from build123d import *

# Parameters (mm, degrees)
BOSS_EXTRUDE1_DEPTH = 4.95
CUT_EXTRUDE1_DEPTH  = 3.45
CUT_EXTRUDE2_REACH  = 63.277
SKETCH3_R           = 0.975
CUT_EXTRUDE3_REACH  = 63.319
SKETCH4_R           = 1.125


with BuildPart() as part:
    # Sketch1 → Boss-Extrude1 (new body)
    with BuildSketch(Plane(origin=(69.394235316, 0, 69.394235316), x_dir=(0.7071067811865475, 0, -0.7071067811865477), z_dir=(0.7071067811865477, 0, 0.7071067811865475))):
        with BuildLine():
            Line((23.501825189, 8.05), (23.501825189, 14.369504832))
            ThreePointArc((23.501825189, 14.369504832), (21.501825189, 17.5), (23.501825189, 20.630495168))
            Line((23.501825189, 20.630495168), (23.501825189, 26.95))
            ThreePointArc((23.501825189, 26.95), (24.380504846, 29.071320344), (26.501825189, 29.95))
            Line((26.501825189, 29.95), (33.522833629, 29.95))
            ThreePointArc((33.522833629, 29.95), (35.951825189, 30.95), (38.38081675, 29.95))
            Line((38.38081675, 29.95), (45.401825189, 29.95))
            ThreePointArc((45.401825189, 29.95), (47.523145533, 29.071320344), (48.401825189, 26.95))
            Line((48.401825189, 26.95), (48.401825189, 20.630495168))
            ThreePointArc((48.401825189, 20.630495168), (50.401825189, 17.5), (48.401825189, 14.369504832))
            Line((48.401825189, 14.369504832), (48.401825189, 8.05))
            ThreePointArc((48.401825189, 8.05), (47.523145533, 5.928679656), (45.401825189, 5.05))
            Line((45.401825189, 5.05), (38.38081675, 5.05))
            ThreePointArc((38.38081675, 5.05), (35.951825189, 4.05), (33.522833629, 5.05))
            Line((33.522833629, 5.05), (26.501825189, 5.05))
            ThreePointArc((26.501825189, 5.05), (24.380504846, 5.928679656), (23.501825189, 8.05))
        make_face()
    extrude(amount=BOSS_EXTRUDE1_DEPTH)

    # Sketch2 → Cut-Extrude1 (cut)
    with BuildSketch(Plane(origin=(72.894413883, 0, 72.894413883), x_dir=(0.7071067811865476, 0, -0.7071067811865476), z_dir=(0.7071067811865476, 0, 0.7071067811865476))):
        with BuildLine():
            Line((38.360144105, 27.95), (46.401825189, 27.95))
            Line((46.401825189, 27.95), (46.401825189, 19.908318916))
            ThreePointArc((46.401825189, 19.908318916), (43.501825189, 17.5), (46.401825189, 15.091681084))
            Line((46.401825189, 15.091681084), (46.401825189, 7.05))
            Line((46.401825189, 7.05), (38.360144105, 7.05))
            ThreePointArc((38.360144105, 7.05), (35.951825189, 5.05), (33.543506273, 7.05))
            Line((33.543506273, 7.05), (25.501825189, 7.05))
            Line((25.501825189, 7.05), (25.501825189, 15.091681084))
            ThreePointArc((25.501825189, 15.091681084), (28.401825189, 17.5), (25.501825189, 19.908318916))
            Line((25.501825189, 19.908318916), (25.501825189, 27.95))
            Line((25.501825189, 27.95), (33.543506273, 27.95))
            ThreePointArc((33.543506273, 27.95), (35.951825189, 29.95), (38.360144105, 27.95))
        make_face()
    extrude(amount=-CUT_EXTRUDE1_DEPTH, mode=Mode.SUBTRACT)

    # Sketch3 → Cut-Extrude2 (cut, up to next)
    with BuildSketch(Plane(origin=(70.454895488, 0, 70.454895488), x_dir=(0.7071067811865475, 0, -0.7071067811865477), z_dir=(0.7071067811865477, 0, 0.7071067811865475)), mode=Mode.PRIVATE) as cut_extrude2_sk1:
        with Locations((35.951825189, 27.5)):
            Circle(SKETCH3_R)
    cut_extrude2_tool1 = extrude(cut_extrude2_sk1.sketch, amount=-CUT_EXTRUDE2_REACH, mode=Mode.PRIVATE) & part.part
    # Sketch3 → Cut-Extrude2 (cut, up to next)
    with BuildSketch(Plane(origin=(70.454895488, 0, 70.454895488), x_dir=(0.7071067811865475, 0, -0.7071067811865477), z_dir=(0.7071067811865477, 0, 0.7071067811865475)), mode=Mode.PRIVATE) as cut_extrude2_sk2:
        with Locations((35.951825189, 7.5)):
            Circle(SKETCH3_R)
    cut_extrude2_tool2 = extrude(cut_extrude2_sk2.sketch, amount=-CUT_EXTRUDE2_REACH, mode=Mode.PRIVATE) & part.part
    add(cut_extrude2_tool1.solids().sort_by_distance((95.876675, 27.5, 45.033116))[0], mode=Mode.SUBTRACT)
    add(cut_extrude2_tool2.solids().sort_by_distance((95.876675, 7.5, 45.033116))[0], mode=Mode.SUBTRACT)

    # Sketch4 → Cut-Extrude3 (cut, up to next)
    with BuildSketch(Plane(origin=(72.894413883, 0, 72.894413883), x_dir=(0.7071067811865476, 0, -0.7071067811865476), z_dir=(0.7071067811865476, 0, 0.7071067811865476)), mode=Mode.PRIVATE) as cut_extrude3_sk1:
        with Locations((24.951825189, 17.5)):
            Circle(SKETCH4_R)
    cut_extrude3_tool1 = extrude(cut_extrude3_sk1.sketch, amount=-CUT_EXTRUDE3_REACH, mode=Mode.PRIVATE) & part.part
    # Sketch4 → Cut-Extrude3 (cut, up to next)
    with BuildSketch(Plane(origin=(72.894413883, 0, 72.894413883), x_dir=(0.7071067811865476, 0, -0.7071067811865476), z_dir=(0.7071067811865476, 0, 0.7071067811865476)), mode=Mode.PRIVATE) as cut_extrude3_sk2:
        with Locations((46.951825189, 17.5)):
            Circle(SKETCH4_R)
    cut_extrude3_tool2 = extrude(cut_extrude3_sk2.sketch, amount=-CUT_EXTRUDE3_REACH, mode=Mode.PRIVATE) & part.part
    add(cut_extrude3_tool1.solids().sort_by_distance((90.538019, 17.5, 55.250809))[0], mode=Mode.SUBTRACT)
    add(cut_extrude3_tool2.solids().sort_by_distance((106.094368, 17.5, 39.69446))[0], mode=Mode.SUBTRACT)


solid = part.part
Read the model definition and answer for the solid it produces. Units are mm, in the model's axes. A direction names the side the tool comes from. Coordinates: 2 decimals unless noted, no trailing zeros. Write each loop counter-clockwise with the first axis right and the second up, starting at its lowest first coordinate (ties: lowest second). Pieces come first, ordered by that corner, then holes. Notation, with made-up numbers: (57, 44.5) -> (116, 44.5) arc R14 ccw to (116, 61.5) -> close; hole circle Ø6 at (-29.5, 18.25). An arc over 180 degrees is marked (long way). Return JSON: item names as keys, results as strings.
(1) The part is cut by section A-A on y = 22. Give the vertices of the cut face in (x, z).
Answers below:
{"outline": "(86.01, 52.78) -> (103.62, 35.17) -> (107.12, 38.67) -> (105.71, 40.08) -> (103.27, 37.64) -> (88.49, 52.42) -> (90.93, 54.86) -> (89.51, 56.28) -> close"}
(2) For a pull along X with two mould halves and no side action, classify faces 6 (the cylindrical face through (106.76, 17.55, 35.48)), 7 (the flat face through (93, 27.95, 51)), 8 (the cylindrical face through (104.796, 18.449, 37.541)) as pulls with the +X half, pulls with the -X half, needs draft (parallel to the pull), parting line crosses it, or undercut.
Answers below:
{"face 6": "pulls with the +X half", "face 7": "needs draft", "face 8": "undercut"}
(3) The part is cut by section B-B on z = 39.25. State how many separate pieces and enclosed holes the cut face has, then the cut area to 3 significant figures.
Answers below:
{"separate pieces": "1", "enclosed holes": "2", "area": "115 mm^2"}
(4) The part is cut by section C-C on y = 29. Give the vertices of the cut face in (x, z).
Answers below:
{"outline": "(86.59, 52.2) -> (103.05, 35.74) -> (106.55, 39.24) -> (99.69, 46.1) -> (97.25, 43.66) -> (94.51, 46.4) -> (96.95, 48.84) -> (90.09, 55.7) -> close"}
(5) Which of the six approach directions +Z, -Z, +X, -X, +Y, -Y give full straight-line access (tool end or side, diameter ignored) to faces 1 (the flat face through (87.738, 11.166, 54.502)), 2 (the flat face through (102, 27.95, 42)), 3 (the flat face through (101, 29.95, 42)), 4 (the flat face through (92, 29.95, 50)), 5 (the cylindrical face through (97.15, 5.05, 46.24))?
Answers below:
{"face 1": "+Z, -X, -Y", "face 2": "+Z", "face 3": "-Z, +X, +Y", "face 4": "+Z, -X, +Y", "face 5": "none"}
(6) Consider line 1 along Y through (x, z) = (100, 45); line 2 along X through (y, z) = (10.5, 40); line 3 along Z through (x, y) = (96.5, 29). Determine where each line is inside the solid, lowest interval first. Write a range as from..to.
Answers below:
{"line 1": "5.05..7.05, 27.95..29.95", "line 2": "98.79..100.91, 105.62..105.79", "line 3": "42.29..44.41, 48.4..49.29"}
(7) Each of these flat-tipped pins is pushed along its axis until it touches: P1, Ø6.5, axis at x = 101, z = 43.5, coming from the -Y side; P2, Ø10, axis at x = 105, z = 54, coming from the +Y side; P3, Ø9.5, axis at x = 94, z = 51.5, coming from the +Y side; P4, Ø12, axis at y = 27, z = 36, coming from the -X side. Where does it stop, or does it pass through?
Answers below:
{"P1": "y = 4.37", "P2": "through", "P3": "y = 30.75", "P4": "x = 96.79"}
